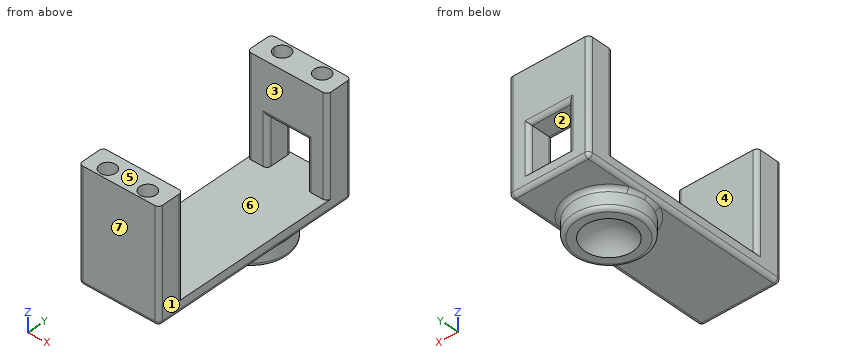
from build123d import *

# Parameters (mm, degrees)
SKETCH1_W           = 20
SKETCH1_H           = 6.65
SKETCH1_H_2         = 20
BOSS_EXTRUDE1_DEPTH = 3
SKETCH1_3_W         = 20
SKETCH1_3_H         = 6.65
BOSS_EXTRUDE2_DEPTH = 25
SKETCH3_R           = 2
CUT_EXTRUDE1_DEPTH  = 5
SKETCH4_R           = 9
BOSS_EXTRUDE3_DEPTH = 5
CUT_EXTRUDE2_REACH  = 64.176
SKETCH6_W           = 5
SKETCH6_H           = 12
FILLET2_R           = 1
FILLET3_R           = 1


with BuildPart() as part:
    # Sketch1 → Boss-Extrude1 (new body)
    with BuildSketch(Plane.XY):
        with Locations((10, 3.325)):
            Rectangle(SKETCH1_W, SKETCH1_H)
        with Locations((10, -10)):
            Rectangle(SKETCH1_W, SKETCH1_H_2)
        with Locations((10, -30)):
            Rectangle(SKETCH1_W, SKETCH1_H_2)
        with Locations((10, -43.325)):
            Rectangle(SKETCH1_W, SKETCH1_H)
    extrude(amount=-BOSS_EXTRUDE1_DEPTH)

    # Sketch1_3 → Boss-Extrude2 (add)
    with BuildSketch(Plane.XY):
        with Locations((10, 3.325)):
            Rectangle(SKETCH1_3_W, SKETCH1_3_H)
        with Locations((10, -43.325)):
            Rectangle(SKETCH1_3_W, SKETCH1_3_H)
    extrude(amount=BOSS_EXTRUDE2_DEPTH)

    # Sketch3 → Cut-Extrude1 (cut)
    with BuildSketch(Plane.XY.offset(25)):
        with BuildLine():
            ThreePointArc((3, 4.15), (3.585786438, 2.735786438), (5, 2.15))
            Line((5, 2.15), (5, 4.15))
            Line((5, 4.15), (3, 4.15))
        make_face()
        with BuildLine():
            Line((5, 4.15), (5, 2.15))
            ThreePointArc((5, 2.15), (6.414213562, 2.735786438), (7, 4.15))
            ThreePointArc((7, 4.15), (5, 6.15), (3, 4.15))
            Line((3, 4.15), (5, 4.15))
        make_face()
        with Locations((15, 4.15)):
            Circle(SKETCH3_R)
        with Locations((5, -44.15)):
            Circle(SKETCH3_R)
        with Locations((15, -44.15)):
            Circle(SKETCH3_R)
    extrude(amount=-CUT_EXTRUDE1_DEPTH, mode=Mode.SUBTRACT)

    # Sketch4 → Boss-Extrude3 (add)
    with BuildSketch(Plane(origin=(0, 0, -3), x_dir=(-1, 0, 0), z_dir=(0, 0, -1))):
        with Locations((-10, -10)):
            Circle(SKETCH4_R)
    extrude(amount=BOSS_EXTRUDE3_DEPTH)

    # Sketch5 → Cut-Revolve1 (revolve, cut)
    with BuildSketch(Plane(origin=(10, 0, 0), x_dir=(0, 0, -1), z_dir=(1, 0, 0)), mode=Mode.PRIVATE) as cut_revolve1_sk:
        with BuildLine():
            ThreePointArc((5, -10), (5.791796068, -6.645898034), (8, -4))
            Line((8, -4), (8, -10))
            Line((8, -10), (5, -10))
        make_face()
    revolve(cut_revolve1_sk.sketch.rotate(Axis((10, -10, -8), (0, 0, 1)), 180), axis=Axis((10, -10, -8), (0, 0, 1)), mode=Mode.SUBTRACT)

    # Sketch6 → Cut-Extrude2 (cut, up to next)
    with BuildSketch(Plane(origin=(0, 6.65, 0), x_dir=(1, 0, 0), z_dir=(0, 1, 0)), mode=Mode.PRIVATE) as cut_extrude2_sk1:
        with Locations((7.5, -6)):
            Rectangle(SKETCH6_W, SKETCH6_H)
    cut_extrude2_tool1 = extrude(cut_extrude2_sk1.sketch, amount=-CUT_EXTRUDE2_REACH, mode=Mode.PRIVATE) & part.part
    # Sketch6 → Cut-Extrude2 (cut, up to next)
    with BuildSketch(Plane(origin=(0, 6.65, 0), x_dir=(1, 0, 0), z_dir=(0, 1, 0)), mode=Mode.PRIVATE) as cut_extrude2_sk2:
        with Locations((12.5, -6)):
            Rectangle(SKETCH6_W, SKETCH6_H)
    cut_extrude2_tool2 = extrude(cut_extrude2_sk2.sketch, amount=-CUT_EXTRUDE2_REACH, mode=Mode.PRIVATE) & part.part
    add(cut_extrude2_tool1.solids().sort_by_distance((7.5, 6.65, 6))[0], mode=Mode.SUBTRACT)
    add(cut_extrude2_tool2.solids().sort_by_distance((12.5, 6.65, 6))[0], mode=Mode.SUBTRACT)

    # Fillet2
    fillet2_edges = [part.edges().sort_by_distance(p)[0] for p in [
        (0, 6.65, 11),
        (20, 6.65, 11),
        (20, -46.65, 11),
        (0, -46.65, 11),
        (10, -46.65, -3),
        (20, -20, -3),
        (0, 0, 12.5),
        (20, 0, 12.5),
        (20, -40, 12.5),
        (0, -40, 12.5),
        (10, 6.65, -3),
        (0, -20, -3),
        (19, -10, -8),
        (10, 6.65, 12),
        (15, 6.65, 6),
        (5, 0, 6),
        (5, 6.65, 6),
        (15, 0, 6),
        (10, 0, 12),
    ]]
    fillet(fillet2_edges, radius=FILLET2_R - 0.0001)  # a hair under: the kernel refuses the full size

    # Fillet3
    fillet3_edges = [part.edges().sort_by_distance(p)[0] for p in [
        (19, -10, -3),
        (19, -10, -3),
    ]]
    fillet(fillet3_edges, radius=FILLET3_R)


solid = part.part
The model under review builds one solid part; all positions refer to its coordinate system, in mm. Face numbers are marked on the shaded views. A direction names the side the tool comes from. Round coordinates to 2 decimals unless told otherwise and drop trailing zeros. Order: outer loops, then holes, each group sorted by start corner. A loop starts at its lowest first (then second) coordinate and runs counter-clockwise, first axis right, second up. Notation, with made-up numbers: (-8.5, 85) -> (40.5, 85) arc R20 ccw to (40.5, 121) -> close; hole circle Ø1 at (63, 41.25). An arc over 180 degrees is marked (long way). Use CSV: the item, a comma, the result in double quotes. Start each with the question number.
(1) Consider section A-A on z = 15.5. Write out the cut boundary in (x, y), and give its area (3 significant figures).
(2) Insertion check: pin 1 (3 mm diameter, centred on x = 15, y = -44.15, fed in from -Z); pin 2 (10 mm diameter, centred on x = 18, y = -22.5, fed in from +Z); pin 3 (8 mm diameter, centred on x = 4.5, z = 3.5, fed in from +Y); pin 4 (1.2 mm diameter, centred on x = 6, y = -44.5, fed in from +Z). Each pin has a flat end and moves straight along its axis. Give the tip position at first contact, or say it passes through.
(3) Tool access review of the marked faces 1, 2 and 3: name each direction out of +Z, -Z, +X, -X, +Y, -Y from which nothing blocks a thin tool from reaching the whole face with its end or side.
(4) Consider section C-C on x = 10. Write out the cut boundary in (y, z).
(5) Wall thickness on probe 1 along X at (y, z) = (4, 23); probe 2 along Y at (x, z) = (5, 22); probe 3 along Y at (x, z) = (1, 7): over which ranges is each line inside the solid? List them lowest first. Write a range as from..to.
(6) Mouldability with a two-part tool opening along Y and no side actions: class the marked faces 4, 5, 6 and 7 as pulls with the +Y half, pulls with the -Y half, needs draft (parallel to the pull), parting line crosses it, or undercut.
(7) Consider section D-D on z = 9. Write out the cut boundary in (x, y), and give its area (3 significant figures).
(8) Consider section B-B on z = 22.5. Write out the cut boundary in (x, y), and give its area (3 significant figures).
Responses:
1,outline,"(0, -45.65) arc R1 ccw to (1, -46.65) -> (19, -46.65) arc R1 ccw to (20, -45.65) -> (20, -41) arc R1 ccw to (19, -40) -> (1, -40) arc R1 ccw to (0, -41) -> close; (0, 1) arc R1 ccw to (1, 0) -> (19, 0) arc R1 ccw to (20, 1) -> (20, 5.65) arc R1 ccw to (19, 6.65) -> (1, 6.65) arc R1 ccw to (0, 5.65) -> close"
1,area,"264 mm²"
2,pin 1,"z = -3"
2,pin 2,"z = 0"
2,pin 3,"y = 6.65"
2,pin 4,"z = 20"
3,face 1,"+Z, -Z, +X, +Y, -Y"
3,face 2,"+Y"
3,face 3,"+Z, +X, -X"
4,outline,"(-46.65, -2) arc R1 ccw to (-45.65, -3) -> (-20, -3) arc R1 cw to (-19, -4) -> (-19, -7) arc R1 ccw to (-18, -8) -> (-16, -8) arc R7.5 cw to (-4, -8) -> (-2, -8) arc R1 ccw to (-1, -7) -> (-1, -4) arc R1 cw to (0, -3) -> (5.65, -3) arc R1 ccw to (6.65, -2) -> (6.65, 0) -> (-40, 0) -> (-40, 25) -> (-46.65, 25) -> close; (0, 13) arc R1 ccw to (1, 12) -> (5.65, 12) arc R1 ccw to (6.65, 13) -> (6.65, 25) -> (0, 25) -> close"
5,probe 1,"0..3.01, 6.99..13.01, 16.99..20"
5,probe 2,"-46.65..-46.15, -42.15..-40, 0..2.15, 6.15..6.65"
5,probe 3,"-46.65..-40, 0..6.65"
6,face 4,"undercut"
6,face 5,"needs draft"
6,face 6,"undercut"
6,face 7,"pulls with the -Y half"
7,outline,"(0, -45.65) arc R1 ccw to (1, -46.65) -> (19, -46.65) arc R1 ccw to (20, -45.65) -> (20, -41) arc R1 ccw to (19, -40) -> (1, -40) arc R1 ccw to (0, -41) -> close; (0, 1) arc R1 ccw to (1, 0) -> (4, 0) arc R1 ccw to (5, 1) -> (5, 5.65) arc R1 ccw to (4, 6.65) -> (1, 6.65) arc R1 ccw to (0, 5.65) -> close; (15, 1) arc R1 ccw to (16, 0) -> (19, 0) arc R1 ccw to (20, 1) -> (20, 5.65) arc R1 ccw to (19, 6.65) -> (16, 6.65) arc R1 ccw to (15, 5.65) -> close"
7,area,"197 mm²"
8,outline,"(0, -45.65) arc R1 ccw to (1, -46.65) -> (19, -46.65) arc R1 ccw to (20, -45.65) -> (20, -41) arc R1 ccw to (19, -40) -> (1, -40) arc R1 ccw to (0, -41) -> close; (0, 1) arc R1 ccw to (1, 0) -> (19, 0) arc R1 ccw to (20, 1) -> (20, 5.65) arc R1 ccw to (19, 6.65) -> (1, 6.65) arc R1 ccw to (0, 5.65) -> close; hole circle Ø4 at (5, -44.15); hole circle Ø4 at (5, 4.15); hole circle Ø4 at (15, -44.15); hole circle Ø4 at (15, 4.15)"
8,area,"214 mm²"
